Design review of the part built by this model. Coordinates are the model's own, in mm. A direction names the side the tool comes from. Coordinates: 2 decimals unless noted, no trailing zeros. Write each loop counter-clockwise with the first axis right and the second up, starting at its lowest first coordinate (ties: lowest second). Pieces come first, ordered by that corner, then holes.
Q1. The part is to be moulded in two halves that separate along X. For faces 4 (the face through (-11, 0, 26)), 5 (the face through (-8.155, -0.049, 22.618)), 6 (the face through (12.932, -5.362, 12.413)), 7 (the face through (-3, 10, 0)), say which applies: +X half, -X half, draft (parallel to the pull), parting line (faces both ways), or undercut.
Q2. Add section A-A, the plane y = 0. Give the boundary of the cut face in (x, z), plus the area to 3 significant figures.
Q3. To check wall thickness, follow probe 1 along Y at (x, z) = (0, 15.5); probe 2 along X at (y, z) = (4.25, 29.5); probe 3 along Y at (x, z) = (-4, 2.5). State the ranges of each line that lie inside material, in increasing order.
Q4. Clearance check with flat-ended pins moving along their axes: pin 1 Ø2 at (x, z) = (4, 20.5) entering from -Y; pin 2 Ø5 at (x, y) = (-9, -11.5) entering from +Z; pin 3 Ø1 at (y, z) = (4, 24) entering from +X. State where each tip first meets the part, or that it passes through.
Q5. Add section D-D, the plane y = -4. Give the boundary of the cut face in (x, z).
Q6. Machinability: for faces 1 (the face through (0.1, -3.5, 22.8)), 2 (the face through (-7, 10, 24)), 3 (the face through (9, -7.5, 26)), which of the approach directions +Z, -Z, +X, -X, +Y, -Y give a long, thin tool a straight path to every point of the face, cutting with its end or side? Answer none if there is none.
Q7. Add section C-C, the plane z = 22.5. Give the boundary of the cut face in (x, y).
Q8. Add section B-B, the plane x = 0. Give the boundary of the cut face in (y, z).
from build123d import *

# Parameters (mm, degrees)
CYLINDER001_R               = 11
CYLINDER001_DEPTH           = 7
CYLINDER001_ROLL_ANGLE      = 90
CYLINDER001_PLACEMENT_ANGLE = 180
CYLINDER003_R               = 7
CYLINDER003_DEPTH           = 30
CYLINDER003_ROLL_ANGLE      = -90
BOX001_W                    = 30
BOX001_H                    = 10
BOX001_DEPTH                = 6
BOX002_W                    = 30
BOX002_H                    = 10
BOX002_DEPTH                = 6
CYLINDER_R                  = 10
CYLINDER_DEPTH              = 20
PAD001_DEPTH                = 14
PAD001_DEPTH_BACK           = -14
CYLINDER002_R               = 14
CYLINDER002_DEPTH           = 30


with BuildPart() as bearing:
    # Cylinder001 → Cylinder001 (new body)
    with BuildSketch(Plane.XY):
        Circle(CYLINDER001_R)
    extrude(amount=CYLINDER001_DEPTH)


with BuildPart() as bearing_1:
    # Cylinder001 roll: moved
    add(bearing.part.rotate(Axis((0, 0, 0), (1, 0, 0)), CYLINDER001_ROLL_ANGLE))


with BuildPart() as bearing_2:
    # Cylinder001 placement: moved
    add(bearing_1.part.moved(Location((0, -3.5, 30))).rotate(Axis((0, -3.5, 30), (0, 0, 1)), CYLINDER001_PLACEMENT_ANGLE))


with BuildPart() as cylinder001:
    # Cylinder003 → Cylinder003 (new body)
    with BuildSketch(Plane.XY):
        Circle(CYLINDER003_R)
    extrude(amount=CYLINDER003_DEPTH)


with BuildPart() as cylinder001_1:
    # Cylinder003 roll: moved
    add(cylinder001.part.rotate(Axis((0, 0, 0), (1, 0, 0)), CYLINDER003_ROLL_ANGLE))


with BuildPart() as cylinder001_2:
    # Cylinder003 placement: moved
    add(cylinder001_1.part.moved(Location((0, -15, 30))))


with BuildPart() as cube001:
    # Box001 → Box001 (new body)
    with BuildSketch(Plane(origin=(-15, -17.5, 24), x_dir=(1, 0, 0), z_dir=(0, 0, 1))):
        with Locations((15, 5)):
            Rectangle(BOX001_W, BOX001_H)
    extrude(amount=BOX001_DEPTH)


with BuildPart() as cube002:
    # Box002 → Box002 (new body)
    with BuildSketch(Plane(origin=(-15, 7.5, 24), x_dir=(1, 0, 0), z_dir=(0, 0, 1))):
        with Locations((15, 5)):
            Rectangle(BOX002_W, BOX002_H)
    extrude(amount=BOX002_DEPTH)


with BuildPart() as negative_fusion:
    # Cylinder → Cylinder (new body)
    with BuildSketch(Plane.XY):
        Circle(CYLINDER_R)
    extrude(amount=CYLINDER_DEPTH)

    # Fusion: union Bearing, Cylinder001, Cube001, Cube002
    add(bearing_2.part)
    add(cylinder001_2.part)
    add(cube001.part)
    add(cube002.part)


with BuildPart() as body001:
    # Sketch001 → Pad001 (new body, two sides)
    with BuildSketch(Plane.XZ) as pad001_sk:
        Polygon((-7, 0), (7, 0), (15, -8), (15, -30), (-15, -30), (-15, -8), align=None)
    extrude(amount=-PAD001_DEPTH)
    extrude(pad001_sk.sketch, amount=-PAD001_DEPTH_BACK)


with BuildPart() as body001_1:
    # Body001 placement: moved
    add(body001.part.moved(Location((0, 0, 30))))


with BuildPart() as cut:
    # Cylinder002 → Cylinder002 (new body)
    with BuildSketch(Plane.XY):
        Circle(CYLINDER002_R)
    extrude(amount=CYLINDER002_DEPTH)

    # Common: intersect Body001
    add(body001_1.part, mode=Mode.INTERSECT)

    # Cut: cut Negative Fusion
    add(negative_fusion.part, mode=Mode.SUBTRACT)


solid = cut.part
Here are the results:
1. face 4: -X half
1. face 5: undercut
1. face 6: parting line
1. face 7: draft
2. outline: (-14, 0) - (-10, 0) - (-10, 20) - (-4.58, 20) arc R11 cw to (-10.45, 26.55) - (-14, 23) - close; (4.58, 20) - (10, 20) - (10, 0) - (14, 0) - (14, 23) - (10.45, 26.55) arc R11 cw to start
2. area: 222 mm2
3. probe 1: y = -14 to -10, 10 to 14
3. probe 2: x = -7.5 to -6.98, 6.98 to 7.5
3. probe 3: y = -13.42 to -9.17, 9.17 to 13.42
4. pin 1: stops at y = -13.67
4. pin 2: stops at z = 24
4. pin 3: stops at x = 13.47
5. outline: (-13.42, 0) - (-9.17, 0) - (-9.17, 20) - (9.17, 20) - (9.17, 0) - (13.42, 0) - (13.42, 23.58) - (7, 30) arc R7 cw to (-7, 30) - (-13.42, 23.58) - close
6. face 1: +Z
6. face 2: +Z, +X, -X, +Y
6. face 3: +Z, +X, -X, -Y
7. outline: circle Ø28 at (0, 0); hole (-8.05, -3.5) - (8.05, -3.5) - (8.05, 3.5) - (-8.05, 3.5) - close
8. outline: (-14, 0) - (-10, 0) - (-10, 20) - (-3.5, 20) - (-3.5, 23) - (-14, 23) - close; (3.5, 20) - (10, 20) - (10, 0) - (14, 0) - (14, 23) - (3.5, 23) - close
